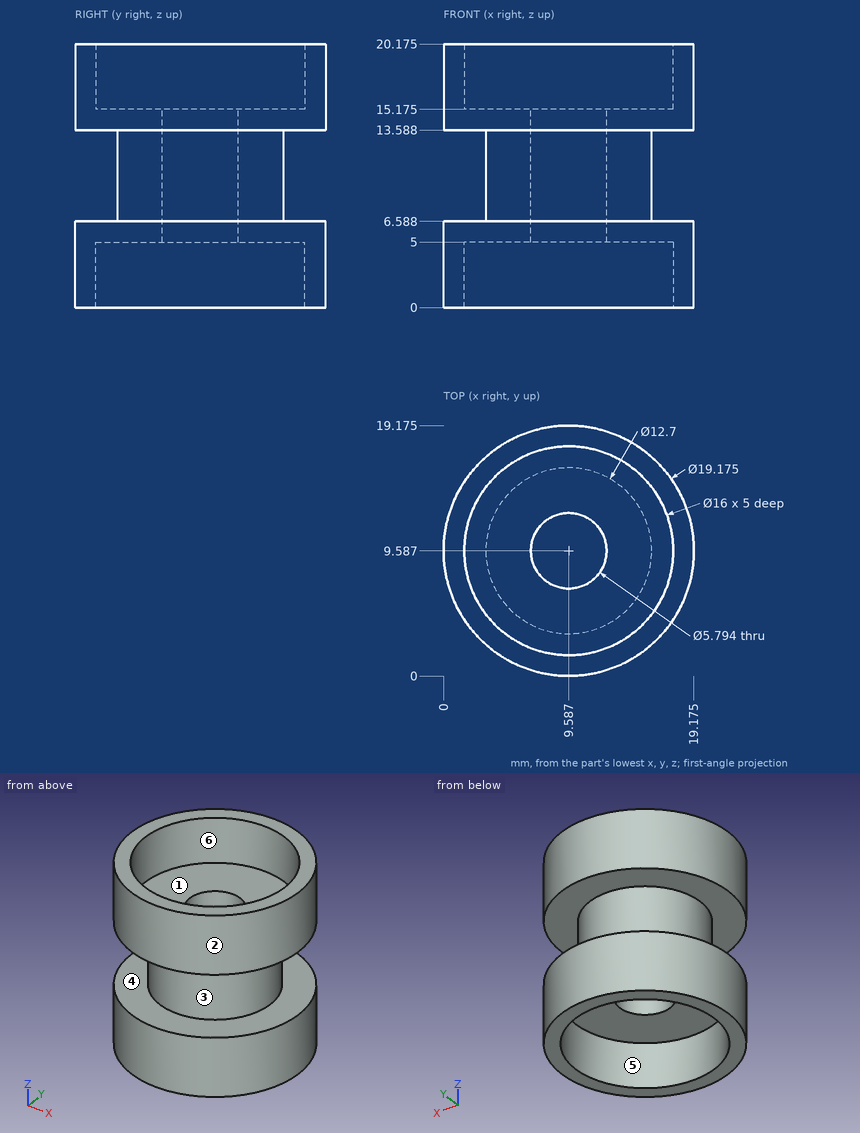
Print and shaded views of the part. All mm, measured from the part's lowest x, y and z. A direction names the side the tool comes from. Give positions to 0.01 mm unless a question says otherwise; leave off trailing zeros.
1) Flat gauge pins, fed straight in: pin 1 Ø10 at (y, z) = (2, 16) entering from -X (1 decimal); pin 2 Ø5 at (x, y) = (11.5, 6.5) entering from +Z (1 decimal); pin 3 Ø1 at (y, z) = (16, 2.5) entering from -X. Where does each tip first touch, or does it go through?
2) Pull direction Z, two halves, no side cores. Call the marked faces 1, 2 and 3: +Z half, -Z half, draft (parallel to the pull), parting line (faces both ways), or undercut.
3) Wall check: line 1 (Z direction, x = 3, y = 7) (1 decimal); line 2 (Z direction, x = 13.25, y = 1.75) (1 decimal); line 3 (Z direction, x = 14.25, y = 9.25) (1 decimal). Give the ranges that are in metal, low to high.
4) Tool access for the marked faces 4, 5 and 6: list every direction of +Z, -Z, +X, -X, +Y, -Y with a clear straight run to the whole face (end or side of a thin tool).
Answer block:
1. pin 1: stops at x = 0.4
1. pin 2: stops at z = 15.2
1. pin 3: stops at x = 2.04
2. face 1: +Z half
2. face 2: draft
2. face 3: undercut
3. line 1: z = 5 to 6.6, 13.6 to 15.2
3. line 2: z = 0 to 6.6, 13.6 to 20.2
3. line 3: z = 5 to 15.2
4. face 4: none
4. face 5: -Z
4. face 6: +Z
